Model file for the job. Use its own axes, mm. A direction names the side the tool comes from. Give positions to 0.01 mm unless a question says otherwise; leave off trailing zeros. Loops run counter-clockwise (first coordinate to the right, second up) from the corner with the lowest first, then second, coordinate; pieces in that order, holes last. Notation, with made-up numbers: M 17,-0.75 L 55,-0.75 A32 cw 55,28.25 Z; hole C -28.75,47 d10. An arc over 180 degrees is marked long. Answer in a Markdown table with one row per item.
```python
from build123d import *

# Parameters (mm, degrees)
SKETCH039_W                                      = 30
SKETCH039_H                                      = 15
SKETCH039_R                                      = 1.6
PAD008_DEPTH                                     = 5
SKETCH040_W                                      = 4.5
SKETCH040_H                                      = 2.8
SKETCH040_W_2                                    = 5.5
SKETCH040_W_3                                    = 2.8
SKETCH040_H_2                                    = 5.5
PAD009_DEPTH                                     = 1
PAD010_DEPTH                                     = 1
FILLET002_R                                      = 1
CHAMFER004013007011015006009007001005003045_SIZE = 0.4
CHAMFER004013007011015006009007001005003046_SIZE = 0.4


with BuildPart() as part:
    # Sketch039 → Pad008 (new body)
    with BuildSketch(Plane.XY):
        with Locations((15, 7.5)):
            Rectangle(SKETCH039_W, SKETCH039_H)
        with Locations((7.5, 7.5)):
            Circle(SKETCH039_R, mode=Mode.SUBTRACT)
        with Locations((22.5, 7.5)):
            Circle(SKETCH039_R, mode=Mode.SUBTRACT)
    extrude(amount=PAD008_DEPTH)

    # Sketch040 (on Face8 of Pad008) → Pad009 (join)
    with BuildSketch(Plane.XY.offset(5)):
        with Locations((18.25, 7.5)):
            Rectangle(SKETCH040_W, SKETCH040_H)
        with Locations((27.25, 7.5)):
            Rectangle(SKETCH040_W_2, SKETCH040_H)
        with Locations((7.5, 12.25)):
            Rectangle(SKETCH040_W_3, SKETCH040_H_2)
        with Locations((7.5, 2.75)):
            Rectangle(SKETCH040_W_3, SKETCH040_H_2)
    extrude(amount=PAD009_DEPTH)

    # Sketch040 (on Face8 of Pad008) → Pad010 (join)
    with BuildSketch(Plane.XY.offset(5)):
        with Locations((18.25, 7.5)):
            Rectangle(SKETCH040_W, SKETCH040_H)
        with Locations((27.25, 7.5)):
            Rectangle(SKETCH040_W_2, SKETCH040_H)
        with Locations((7.5, 12.25)):
            Rectangle(SKETCH040_W_3, SKETCH040_H_2)
        with Locations((7.5, 2.75)):
            Rectangle(SKETCH040_W_3, SKETCH040_H_2)
    extrude(amount=PAD010_DEPTH)

    # Fillet002
    fillet002_edges = [part.edges().sort_by_distance(p)[0] for p in [
        (30, 0, 2.5),
        (30, 15, 2.5),
        (0, 15, 2.5),
        (0, 0, 2.5),
    ]]
    fillet(fillet002_edges, radius=FILLET002_R)

    # Chamfer004013007011015006009007001005003045
    chamfer004013007011015006009007001005003045_edges = [part.edges().sort_by_distance(p)[0] for p in [
        (30, 8.9, 5.5),
        (24.5, 8.9, 5.5),
        (20.5, 8.9, 5.5),
        (16, 8.9, 5.5),
        (16, 6.1, 5.5),
        (8.9, 15, 5.5),
        (6.1, 15, 5.5),
        (8.9, 5.5, 5.5),
        (6.1, 5.5, 5.5),
        (6.1, 9.5, 5.5),
        (6.1, 0, 5.5),
        (8.9, 9.5, 5.5),
        (8.9, 0, 5.5),
        (20.5, 6.1, 5.5),
        (24.5, 6.1, 5.5),
        (30, 6.1, 5.5),
    ]]
    chamfer(chamfer004013007011015006009007001005003045_edges, length=CHAMFER004013007011015006009007001005003045_SIZE)

    # Chamfer004013007011015006009007001005003046
    chamfer004013007011015006009007001005003046_edges = [part.edges().sort_by_distance(p)[0] for p in [
        (15, 0, 0),
        (29.707107, 0.292893, 0),
        (30, 7.5, 0),
        (29.707107, 14.707107, 0),
        (15, 15, 0),
        (0.292893, 14.707107, 0),
        (0, 7.5, 0),
        (0.292893, 0.292893, 0),
        (20.9, 7.5, 0),
        (5.9, 7.5, 0),
    ]]
    chamfer(chamfer004013007011015006009007001005003046_edges, length=CHAMFER004013007011015006009007001005003046_SIZE)


solid = part.part
```
(1) Saw through at C-C, the plane y = 7.5. Give the cut face in (x, z), and give its area (3 significant figures).
Established:
| item | result |
|---|---|
| outline | M 0,0.4 L 0.4,0 L 5.5,0 L 5.9,0.4 L 5.9,5 L 0,5 Z; M 9.1,0.4 L 9.5,0 L 20.5,0 L 20.9,0.4 L 20.9,5 L 20.5,5 L 20.5,6 L 16,6 L 16,5 L 9.1,5 Z; M 24.1,0.4 L 24.5,0 L 29.6,0 L 30,0.4 L 30,6 L 24.5,6 L 24.5,5 L 24.1,5 Z |
| area | 128 mm2 |
(2) Which spindle directions (+Z, -Z, +X, -X, +Y, -Y) get a long thin tool onto all of the face, cutting with end or side? Do faces 1 (the flat face through (27.2, 8.9, 5.5)), 2 (the flat face through (27.2, 6.1, 5.5)), 3 (the flat face through (18, 8, 6)), 4 (the flat face through (7.5, 9.5, 5.5)), 5 (the flat face through (24.5, 7.5, 5.5)). Say none if no direction does.
Established:
| item | result |
|---|---|
| face 1 | +Z, +X, -X, +Y |
| face 2 | +Z, +X, -X, -Y |
| face 3 | +Z, +X, -X, +Y, -Y |
| face 4 | +Z, +X, -X |
| face 5 | +Z, +Y, -Y |
(3) Mould opens along Y. For faces 6 (the conical face through (0.458, 0.47, 0.158)), 7 (the cylindrical face through (7.15, 5.94, 2.67)), 8 (the flat face through (27, 8, 6)) say: pulls with the +Y half, pulls with the -Y half, needs draft (parallel to the pull), parting line crosses it, or undercut.
Established:
| item | result |
|---|---|
| face 6 | pulls with the -Y half |
| face 7 | undercut |
| face 8 | needs draft |
(4) Saw through at A-A, the plane x = 7.5. Give the cut face in (y, z).
Established:
| item | result |
|---|---|
| outline | M 0,0.4 L 0.4,0 L 5.5,0 L 5.9,0.4 L 5.9,5 L 5.5,5 L 5.5,6 L 0,6 Z; M 9.1,0.4 L 9.5,0 L 14.6,0 L 15,0.4 L 15,6 L 9.5,6 L 9.5,5 L 9.1,5 Z |
(5) Saw through at D-D, the plane z = 3. Give the cut face in (x, y), and give its area (3 significant figures).
Established:
| item | result |
|---|---|
| outline | M 0,1 A1 ccw 1,0 L 29,0 A1 ccw 30,1 L 30,14 A1 ccw 29,15 L 1,15 A1 ccw 0,14 Z; hole C 7.5,7.5 d3.2; hole C 22.5,7.5 d3.2 |
| area | 433 mm2 |
(6) Flat gauge pins, fed straight in: P1, Ø0.8, axis at y = 7.5, z = 5.5, coming from the -X side; P2, Ø0.8, axis at x = 28, z = 5.5, coming from the +Y side; P3, Ø2.5, axis at x = 7.5, y = 7.5, coming from the +Z side; P4, Ø0.5, axis at y = 11, z = 5.5, coming from the +X side. Where does each tip first touch, or does it go through?
Established:
| item | result |
|---|---|
| P1 | stops at x = 16 |
| P2 | stops at y = 8.9 |
| P3 | passes through |
| P4 | stops at x = 8.9 |
(7) Saw through at B-B, the plane z = 5.5. Count the separate pieces of the cut face and the enclosed holes in it, and give its area (3 significant figures).
Established:
| item | result |
|---|---|
| separate pieces | 4 |
| enclosed holes | 0 |
| area | 57.5 mm2 |
(8) Wall check: L1, parallel to Y at x = 22.5, z = 2.4; L2, parallel to X at y = 6.25, z = 3.75; L3, parallel to Z at x = 10.5, y = 10.5. Give the ranges that are in metal, low to high.
Established:
| item | result |
|---|---|
| L1 | y = 0 to 5.9, 9.1 to 15 |
| L2 | x = 0 to 6.5, 8.5 to 21.5, 23.5 to 30 |
| L3 | z = 0 to 5 |
